Geometry: final body of the model. Coordinates: model frame, mm. Face numbers are marked on the shaded views. Coordinates: 2 decimals unless noted, no trailing zeros. Order: outer loops, then holes, each group sorted by start corner. A loop starts at its lowest first (then second) coordinate and runs counter-clockwise, first axis right, second up. Notation, with made-up numbers: (56.5, 88.25) -> (66.5, 88.25) arc R31 ccw to (66.5, 116.25) -> close; hole circle Ø1 at (54.25, 81.25). An arc over 180 degrees is marked (long way). Use one line per item in the form item = value.
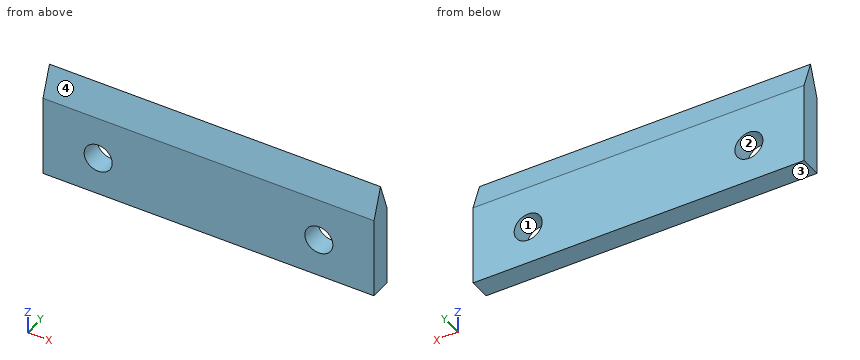
```python
from build123d import *

# Parameters (mm, degrees)
SKETCH_1_W          = 39
SKETCH_1_H          = 13
SKETCH_1_R          = 1.65
EXTRUDE_1_DEPTH     = 2.5
CUT_EXTRUDE_1_DEPTH = 42
CUT_EXTRUDE_2_DEPTH = 42


with BuildPart() as part:
    # 草图1 → 凸台-拉伸1 (new body)
    with BuildSketch(Plane(origin=(0, 0, 0), x_dir=(1, 0, 0), z_dir=(0, 1, 0))):
        with Locations((19.5, 6.5)):
            Rectangle(SKETCH_1_W, SKETCH_1_H)
        with Locations(Location((6.5, 8.5, 0), (0, 0, 270))):
            Circle(SKETCH_1_R, mode=Mode.SUBTRACT)
        with Locations(Location((32.5, 8.5, 0), (0, 0, 270))):
            Circle(SKETCH_1_R, mode=Mode.SUBTRACT)
    extrude(amount=EXTRUDE_1_DEPTH)

    # 草图2 → 切除-拉伸1 (cut)
    with BuildSketch(Plane(origin=(39, 0, 0), x_dir=(0, 0, -1), z_dir=(1, 0, 0))):
        Polygon((3.5, 2.5), (0, 2.5), (0, 1.25), align=None)
    extrude(amount=-CUT_EXTRUDE_1_DEPTH, mode=Mode.SUBTRACT)

    # 草图3 → 切除-拉伸2 (cut)
    with BuildSketch(Plane(origin=(39, 0, 0), x_dir=(0, 0, -1), z_dir=(1, 0, 0))):
        Polygon((0, 1.25), (0, 0), (3.5, 0), align=None)
    extrude(amount=-CUT_EXTRUDE_2_DEPTH, mode=Mode.SUBTRACT)


solid = part.part
```
1) Section C-C, the plane z = -8.5. Output: boundary loops of the cut face in (x, y), and give its area (3 significant figures).
Results found:
outline = (0, 0) -> (4.85, 0) -> (4.85, 2.5) -> (0, 2.5) -> close; (8.15, 0) -> (30.85, 0) -> (30.85, 2.5) -> (8.15, 2.5) -> close; (34.15, 0) -> (39, 0) -> (39, 2.5) -> (34.15, 2.5) -> close
area = 81.0 mm2
2) Section A-A, the plane x = 32.5. Output: boundary loops of the cut face in (y, z).
Results found:
outline = (0, -13) -> (2.5, -13) -> (2.5, -10.15) -> (0, -10.15) -> close; (0, -6.85) -> (2.5, -6.85) -> (2.5, -3.5) -> (1.25, 0) -> (0, -3.5) -> close
3) Pull-direction query (Z, two-part tool) for the marked faces 1, 2, 3 and 4; classes: released by +Z, released by -Z, zero draft, split by the parting line, or undercut.
Results found:
face_1 = undercut
face_2 = undercut
face_3 = released by -Z
face_4 = released by +Z
4) Material intervals for probe 1 along X at (y, z) = (0.7, -8.5); probe 2 along Y at (x, z) = (16, -2.5), sorted ascending. Write a range as from..to.
Results found:
probe_1 = 0..4.85, 8.15..30.85, 34.15..39
probe_2 = 0.36..2.14
5) Contact query for flat-ended pins moving along their axis: P1, Ø4.5, axis at x = 32.5, z = -8.5, coming from the -Y side; P2, Ø2, axis at x = 6.5, z = -8.5, coming from the +Y side (3 decimals). Output: stop coordinate, or through.
Results found:
P1 = 0
P2 = through
6) Section B-B, the plane y = 0.7. Output: boundary loops of the cut face in (x, z).
Results found:
outline = (0, -13) -> (39, -13) -> (39, -1.54) -> (0, -1.54) -> close; hole circle Ø3.3 at (6.5, -8.5); hole circle Ø3.3 at (32.5, -8.5)
7) Section D-D, the plane x = 36.5. Output: boundary loops of the cut face in (y, z).
Results found:
outline = (0, -13) -> (2.5, -13) -> (2.5, -3.5) -> (1.25, 0) -> (0, -3.5) -> close
